```python
from build123d import *

# Parameters (mm, degrees)
SKETCH1_W           = 360
SKETCH1_H           = 235
BOSS_EXTRUDE1_DEPTH = 11
FILLET1_R           = 5
SKETCH2_W           = 348.8
SKETCH2_H           = 216.9
CUT_EXTRUDE1_DEPTH  = 2


with BuildPart() as part:
    # Sketch1 → Boss-Extrude1 (new body)
    with BuildSketch(Plane.XY):
        Rectangle(SKETCH1_W, SKETCH1_H)
    extrude(amount=BOSS_EXTRUDE1_DEPTH)

    # Fillet1
    fillet1_edges = [part.edges().sort_by_distance(p)[0] for p in [
        (180, -117.5, 5.5),
        (-180, -117.5, 5.5),
        (-180, 117.5, 5.5),
        (180, 117.5, 5.5),
    ]]
    fillet(fillet1_edges, radius=FILLET1_R)

    # Sketch2 → Cut-Extrude1 (cut)
    with BuildSketch(Plane.XY.offset(11)):
        with Locations((0, 3.45)):
            Rectangle(SKETCH2_W, SKETCH2_H)
    extrude(amount=-CUT_EXTRUDE1_DEPTH, mode=Mode.SUBTRACT)


solid = part.part
```
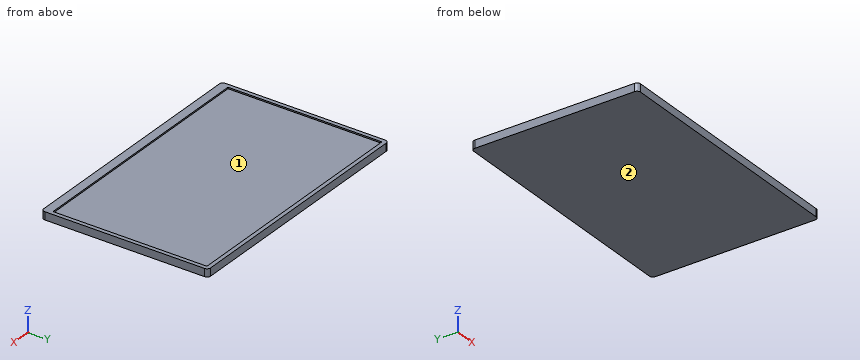
Here's how the part is built. I have some questions about the finished solid (model axes, mm). Face numbers are marked on the shaded views. Round coordinates to 2 decimals unless told otherwise and drop trailing zeros. Loops run counter-clockwise (first coordinate to the right, second up) from the corner with the lowest first, then second, coordinate; pieces in that order, holes last. Notation, with made-up numbers: (23.25, 71) -> (51.25, 71) arc R15 cw to (51.25, 90) -> close; hole circle Ø4 at (77, 55). An arc over 180 degrees is marked (long way). Answer as CSV lines item,"result". Start each with the question number.
1. If we mould it in two halves opening along Y, with no side actions, what happens to the marked faces 1 and 2? For each: pulls with the +Y half, pulls with the -Y half, needs draft (parallel to the pull), parting line crosses it, or undercut.
2. Imagine slicing it at B-B on x = -35.5. Write out the boundary of the cut face in (y, z), plus the area to 3 significant figures.
3. I need wall thicknesses on probe 1 along Y at (x, z) = (-66, 10.25); probe 2 along X at (y, z) = (20, 9.5); probe 3 along Z at (x, y) = (-51, 66). Which ranges of each line are inside material? Lowest first, please. Write a range as from..to.
4. I'm going to push a flat-ended pin straight in: P1, Ø2, axis at x = 49, y = -53, coming from the +Z side. Where does the tip first touch, or does it pass through?
5. Imagine slicing it at A-A on y = 52. Write out the boundary of the cut face in (x, z).
Solution:
1,face 1,"undercut"
1,face 2,"needs draft"
2,outline,"(-117.5, 0) -> (117.5, 0) -> (117.5, 11) -> (111.9, 11) -> (111.9, 9) -> (-105, 9) -> (-105, 11) -> (-117.5, 11) -> close"
2,area,"2,150 mm²"
3,probe 1,"-117.5..-105, 111.9..117.5"
3,probe 2,"-180..-174.4, 174.4..180"
3,probe 3,"0..9"
4,P1,"z = 9"
5,outline,"(-180, 0) -> (180, 0) -> (180, 11) -> (174.4, 11) -> (174.4, 9) -> (-174.4, 9) -> (-174.4, 11) -> (-180, 11) -> close"
